Geometry check sheet. Reference: the model listing, model coordinates, mm. Coordinates: 2 decimals unless noted, no trailing zeros. Loops run counter-clockwise (first coordinate to the right, second up) from the corner with the lowest first, then second, coordinate; pieces in that order, holes last.
Autodesk Inventor part; units mm, degrees
ref_plane "YZ Plane" through (0, 0, 0) normal (1, 0, 0) x (0, 1, 0)
ref_plane "XZ Plane" through (0, 0, 0) normal (0, 1, 0) x (-1, 0, 0)
ref_plane "XY Plane" through (0, 0, 0) normal (0, 0, 1) x (1, 0, 0)
sketch "Sketch1" plane through (0, 0, 0) normal (0, 0, 1) x (1, 0, 0)
  line L0 (0, 0) -> (30.4, 0)
  line L1 (30.4, 0) -> (30.4, 19)
  line L2 (30.4, 19) -> (0, 19)
  line L3 (0, 19) -> (0, 0)
  circle A0 centre (2.5, 2.5) radius 2.5
  circle A1 centre (27.9, 2.5) radius 2.5
  circle A2 centre (2.5, 2.5) radius 1.25
  circle A3 centre (27.9, 2.5) radius 1.25
  dimension "d0" = 30.4
  dimension "d1" = 19
  dimension "d2" = 5
  dimension "d3" = 5
  dimension "d6" = 2.5
  dimension "d7" = 2.5
extrude "Extrusion1" add sketch "Sketch1" along normal blind 0.8
fillet "Fillet1" radius 1 4 edges at (30.4, 0, 0.4) (0, 0, 0.4) (0, 19, 0.4) (30.4, 19, 0.4)
equation "\"d3\" = d2"
properties part number "PCB_Main"
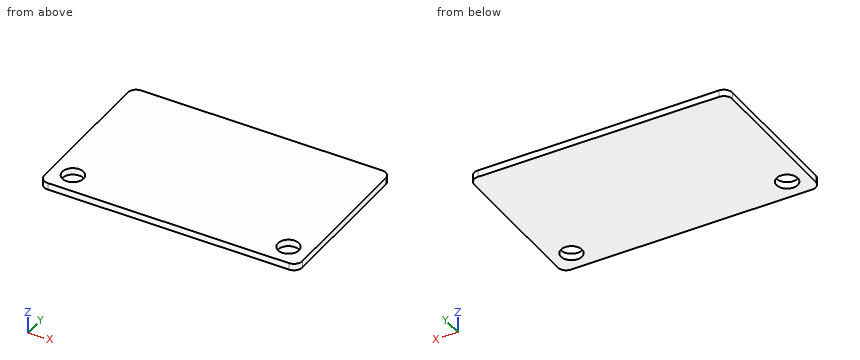
(1) Sectioned sample at C-C on x = 2.5. Record the cut outline in (y, z), and give its area (3 significant figures).
Findings:
outline: (0, 0) - (1.25, 0) - (1.25, 0.8) - (0, 0.8) - close; (3.75, 0) - (19, 0) - (19, 0.8) - (3.75, 0.8) - close
area: 13.2 mm2
(2) Gauge pin test, flat end, axial feed: pin 1 Ø2 at (x, y) = (2.5, 2.5) entering from -Z. Record the tip position at first contact, or that the pin passes through.
Findings:
pin 1: passes through
(3) Sectioned sample at B-B on y = 2.5. Record the cut outline in (x, z).
Findings:
outline: (0, 0) - (1.25, 0) - (1.25, 0.8) - (0, 0.8) - close; (3.75, 0) - (26.65, 0) - (26.65, 0.8) - (3.75, 0.8) - close; (29.15, 0) - (30.4, 0) - (30.4, 0.8) - (29.15, 0.8) - close
(4) Scan lines: L1, parallel to Y at x = 27.9, z = 0.3; L2, parallel to X at y = 2.75, z = 0.7; L3, parallel to Y at x = 2, z = 0.25. Record each from-to range of solid material in increasing order.
Findings:
L1: y = 0 to 1.25, 3.75 to 19
L2: x = 0 to 1.28, 3.72 to 26.68, 29.12 to 30.4
L3: y = 0 to 1.35, 3.65 to 19
(5) Sectioned sample at A-A on z = 0.2. Record the cut outline in (x, y), and give its area (3 significant figures).
Findings:
outline: (0, 1) arc R1 ccw to (1, 0) - (29.4, 0) arc R1 ccw to (30.4, 1) - (30.4, 18) arc R1 ccw to (29.4, 19) - (1, 19) arc R1 ccw to (0, 18) - close; hole circle Ø2.5 at (2.5, 2.5); hole circle Ø2.5 at (27.9, 2.5)
area: 567 mm2
